```python
from build123d import *
from build123d.topology import SkipClean

# Parameters (mm, degrees)
SKETCH2_R                = 12
SKETCH2_R_2              = 10
BOSS_EXTRUDE1_DEPTH      = 2
BOSS_EXTRUDE2_DEPTH      = 70
BOSS_EXTRUDE2_DEPTH_BACK = 2
SKETCH2_2_R              = 10
SKETCH3_R                = 7
CUT_EXTRUDE1_DEPTH       = 74.972968036
SKETCH4_R                = 3
CUT_EXTRUDE2_DEPTH       = 73.027772421
SKETCH4_4_R              = 2
CUT_EXTRUDE3_DEPTH       = 73.027772519
CUT_EXTRUDE4_DEPTH       = 73.027772519
BOSS_EXTRUDE3_DEPTH      = 9
CUT_EXTRUDE5_DEPTH       = 74.972968133
SKETCH6_R                = 2
CUT_EXTRUDE6_DEPTH       = 9


with BuildPart() as part:
    # Sketch2 → Boss-Extrude1 (new body)
    with BuildSketch(Plane(origin=(0, 0, 0), x_dir=(1, 0, 0), z_dir=(0, 1, 0))):
        with Locations(Location((0, 0, 0), (0, 0, 270))):
            Circle(SKETCH2_R)
        with Locations(Location((0, 0, 0), (0, 0, 270))):
            Circle(SKETCH2_R_2, mode=Mode.SUBTRACT)
    extrude(amount=-BOSS_EXTRUDE1_DEPTH)

    # Sketch2<2> → Boss-Extrude2 (add, two sides: drawn at the far end of the back side and taken through both)
    with BuildSketch(Plane(origin=(0, 0, 0), x_dir=(1, 0, 0), z_dir=(0, 1, 0)).offset(-BOSS_EXTRUDE2_DEPTH_BACK)):
        with Locations(Location((0, 0, 0), (0, 0, 270))):
            Circle(SKETCH2_2_R)
    extrude(amount=BOSS_EXTRUDE2_DEPTH + BOSS_EXTRUDE2_DEPTH_BACK)

    # Sketch3 → Cut-Extrude1 (cut, through all)
    with BuildSketch(Plane(origin=(0, 70, 0), x_dir=(1, 0, 0), z_dir=(0, 1, 0))):
        with Locations(Location((0, 0, 0), (0, 0, 270))):
            Circle(SKETCH3_R)
    extrude(amount=-CUT_EXTRUDE1_DEPTH, mode=Mode.SUBTRACT)

    # Sketch4 → Cut-Extrude2 (cut, through all)
    with BuildSketch(Plane.XY):
        with Locations(Location((0, 14, 0), (0, 0, 270))):
            Circle(SKETCH4_R)
    extrude(amount=CUT_EXTRUDE2_DEPTH, mode=Mode.SUBTRACT)

    # Sketch4<4> → Cut-Extrude3 (cut, through all)
    with BuildSketch(Plane.XY):
        with Locations(Location((0, 51, 0), (0, 0, 90))):
            Circle(SKETCH4_4_R)
    extrude(amount=CUT_EXTRUDE3_DEPTH, mode=Mode.SUBTRACT)

    # Sketch4<6> → Cut-Extrude4 (cut, through all)
    with BuildSketch(Plane.XY):
        with BuildLine():
            Line((-2, 44), (-2, 58))
            ThreePointArc((-2, 58), (0, 60), (2, 58))
            Line((2, 58), (2, 44))
            ThreePointArc((2, 44), (0, 42), (-2, 44))
        make_face()
    extrude(amount=CUT_EXTRUDE4_DEPTH, mode=Mode.SUBTRACT)

    # Sketch4<7> → Boss-Extrude3 (add)
    with BuildSketch(Plane.XY):
        with BuildLine():
            Line((-2, 44), (-2, 58))
            ThreePointArc((-2, 58), (0, 60), (2, 58))
            Line((2, 58), (2, 44))
            ThreePointArc((2, 44), (0, 42), (-2, 44))
        make_face()
    extrude(amount=BOSS_EXTRUDE3_DEPTH)

    # Sketch5 → Cut-Extrude5 (cut, through all)
    with BuildSketch(Plane(origin=(0, 70, 0), x_dir=(1, 0, 0), z_dir=(0, 1, 0))):
        with BuildLine():
            Line((3.011686508, -6.318998685), (3.944683927, 2.018210381))
            Line((3.944683927, 2.018210381), (-3.137399774, 2.238378786))
            Line((-3.137399774, 2.238378786), (-2.673709916, -6.469256161))
            ThreePointArc((-2.673709916, -6.469256161), (0.184936128, -6.997556618), (3.011686508, -6.318998685))
        make_face()
    extrude(amount=-CUT_EXTRUDE5_DEPTH, mode=Mode.SUBTRACT)

    # Sketch6 → Cut-Extrude6 (cut)
    with SkipClean():  # the faces are left unmerged after this step: merging them gives an invalid solid
        with BuildSketch(Plane.XY.offset(9)):
            with Locations((0, 51)):
                Circle(SKETCH6_R)
        extrude(amount=-CUT_EXTRUDE6_DEPTH, mode=Mode.SUBTRACT)


solid = part.part
```
Model file for the job. Use its own axes, mm. A direction names the side the tool comes from. Give positions to 0.01 mm unless a question says otherwise; leave off trailing zeros. Loops run counter-clockwise (first coordinate to the right, second up) from the corner with the lowest first, then second, coordinate; pieces in that order, holes last. Notation, with made-up numbers: (33, 73) - (70, 73) arc R27 cw to (70, 112) - close; hole circle Ø10 at (-4.75, -1.75). An arc over 180 degrees is marked (long way). One line per item, written item: value. Start each with the question number.
1. Slice it at B-B (x = -0.75). List the corners of the cut face in (y, z), plus the area to 3 significant figures.
2. Slice it at C-C (y = 27.5). List the corners of the cut face in (x, z), plus the area to 3 significant figures.
3. Pull direction X, two halves, no side cores. Call faces 1 (the flat face through (9, 0, -5)), 2 (the flat face through (0, 46, 9)), 3 (the cylindrical face through (3.604, -0.986, 11.446)): pulls with the +X half, pulls with the -X half, needs draft (parallel to the pull), parting line crosses it, or undercut.
4. Pin check, flat tips, straight feed: pin 1 (5 mm diameter, centred on y = 12.5, z = 4.5, fed in from -X); pin 2 (12.5 mm diameter, centred on x = 0, z = 0, fed in from -Y); pin 3 (2 mm diameter, centred on x = -7.5, y = 55.5, fed in from +Z); pin 4 (4.5 mm diameter, centred on x = 0, y = 46.5, fed in from +Z). Stop position of each tip, or through.
5. Which spindle directions (+Z, -Z, +X, -X, +Y, -Y) get a long thin tool onto all of the face, cutting with end or side? Do faces 4 (the flat face through (-5.2, -2, 5.2)), 5 (the cylindrical face through (-9.76, 34.51, -2.17)), 6 (the cylindrical face through (-2.93, 14.65, 8.14)). Say none if no direction does.
6. Slice it at A-A (z = -1.25). List the corners of the cut face in (x, y), plus the area to 3 significant figures.
7. Probe L1, parallel to Y at x = 0, z = 7.65; L2, parallel to X at y = 28.5, z = 0. List the from-to ranges inside material, lowest first. Write a range as from..to.
8. Slice it at D-D (z = 5). List the corners of the cut face in (x, y), plus the area to 3 significant figures.
Solution:
1. outline: (-2, -11.98) - (0, -11.98) - (0, -9.97) - (70, -9.97) - (70, -6.96) - (-2, -6.96) - close; (-2, 6.96) - (11.1, 6.96) - (11.1, 9.97) - (0, 9.97) - (0, 11.98) - (-2, 11.98) - close; (16.9, 6.96) - (49.15, 6.96) - (49.15, 9) - (42.15, 9) - (42.15, 9.97) - (16.9, 9.97) - close; (52.85, 6.96) - (70, 6.96) - (70, 9.97) - (59.85, 9.97) - (59.85, 9) - (52.85, 9) - close
1. area: 399 mm^2
2. outline: circle Ø20 at (0, 0); hole circle Ø14 at (0, 0)
2. area: 160 mm^2
3. face 1: needs draft
3. face 2: undercut
3. face 3: parting line crosses it
4. pin 1: stops at x = -9.8
4. pin 2: passes through
4. pin 3: stops at z = 7.6
4. pin 4: stops at z = 9.8
5. face 4: +Z, -Z, +X, -X, -Y
5. face 5: +Y
5. face 6: +Z
6. outline: (-11.93, -2) - (-6.89, -2) - (-6.89, 70) - (-9.92, 70) - (-9.92, 0) - (-11.93, 0) - close; (6.89, -2) - (11.93, -2) - (11.93, 0) - (9.92, 0) - (9.92, 70) - (6.89, 70) - close
6. area: 445 mm^2
7. L1: y = -2..11, 17..49, 53..70
7. L2: x = -10..-7, 7..10
8. outline: (-10.91, -2) - (-4.9, -2) - (-4.9, 70) - (-8.66, 70) - (-8.66, 0) - (-10.91, 0) - close; (4.9, -2) - (10.91, -2) - (10.91, 0) - (8.66, 0) - (8.66, 70) - (4.9, 70) - close
8. area: 551 mm^2
